Check sheet for the modelled part. Datum: model origin and axes. Units: mm. Face numbers are marked on the shaded views. A direction names the side the tool comes from. Round coordinates to 2 decimals unless told otherwise and drop trailing zeros. Write each loop counter-clockwise with the first axis right and the second up, starting at its lowest first coordinate (ties: lowest second). Pieces come first, ordered by that corner, then holes. Notation, with made-up numbers: M 39.5,87.25 L 81.5,87.25 A11 cw 81.5,93.25 Z; hole C 13,77 d7. An arc over 180 degrees is marked long. Put each result on its own line as item: value.
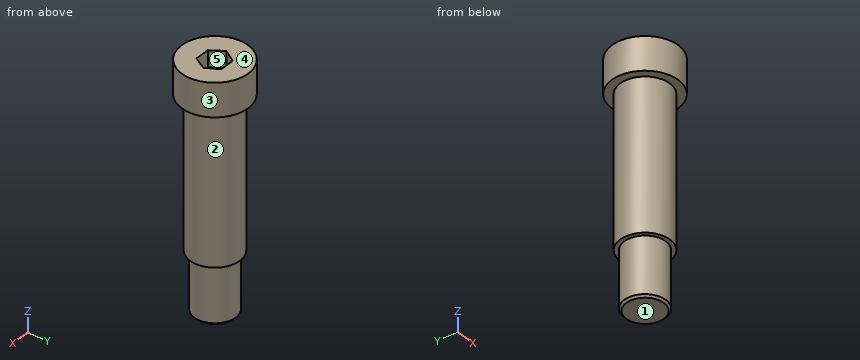
Solid Edge part; units mm, degrees
sketch "Sketch1" plane through (0, 0, 0) normal (0, 0, 1) x (1, 0, 0)
  circle A0 centre (0, 0) radius 12.7
extrude "Protrusion1" add sketch "Sketch1" along normal blind 12.7
sketch "Sketch2" plane through (0, 0, 0) normal (0, 0, -1) x (0, 1, 0)
  circle A0 centre (0, 0) radius 9.525
extrude "Protrusion2" add sketch "Sketch2" along normal blind 57.15
sketch "Sketch3" plane through (0, 0, -57.15) normal (0, 0, -1) x (0, 1, 0)
  circle A0 centre (0, 0) radius 7.9375
extrude "Protrusion3" add sketch "Sketch3" along normal blind 22.225
sketch "Sketch4" plane through (0, 0, 12.7) normal (0, 0, 1) x (0, 1, 0)
  line L0 (-4.7625, 2.6191) -> (0, 5.7431)
  line L1 (-4.7625, -3.0765) -> (-4.7625, 2.6191)
  line L2 (-4.7625, -3.0765) -> (0, -5.7431)
  line L3 (4.7625, -3.0765) -> (0, -5.7431)
  line L4 (4.7625, -3.0765) -> (4.7625, 2.6191)
  line L5 (4.7625, 2.6191) -> (0, 5.7431)
extrude "Cutout1" cut sketch "Sketch4" against normal blind 6.35
chamfer "Chamfer1" distance 0.7874 angle 45 1 edges at (0, -7.9375, -79.375)
properties part number "55030052"
1. Access from +Z, -Z, +X, -X, +Y, -Y to the whole of each face (thin tool, end or side, straight path). Record for the marked faces 1 and 2.
Computed values:
face 1: -Z, +X, -X, +Y, -Y
face 2: -Z
2. Cross-section at C-C (z = -28). Enter the section's corners in (x, y) (3 decimals).
Computed values:
outline: C 0,0 d19.05
3. Cross-section at B-B (z = 2.5). Enter the section's corners in (x, y).
Computed values:
outline: C 0,0 d25.4
4. Release check for a two-part mould opening along X. For the marked faces 3, 4 and 5 record: +X half, -X half, draft (parallel to the pull), parting line (faces both ways), or undercut.
Computed values:
face 3: parting line
face 4: draft
face 5: undercut
5. Depth check by flat-ended pin: pin 1 Ø8 at (x, z) = (-6.5, -58) entering from -Y; pin 2 Ø10 at (y, z) = (-2.5, -20) entering from -X (3 decimals); pin 3 Ø4 at (y, z) = (9.5, -32) entering from +X. Enter the tip coordinate at first touch or a pass-through.
Computed values:
pin 1: stops at y = -9.17
pin 2: stops at x = -9.525
pin 3: stops at x = 5.87
6. Scan lines: probe 1 along Z at (x, y) = (-7.75, 8.5); probe 2 along Z at (x, y) = (-0.75, 3) (3 decimals); probe 3 along Y at (x, z) = (4.5, -31.5). Record each from-to range of solid material in increasing order.
Computed values:
probe 1: z = 0 to 12.7
probe 2: z = -79.375 to 6.35
probe 3: y = -8.39 to 8.39
